Could you check a few things on this drawing? It's one solid part, dimensions in mm from its lowest x, y, z. A direction names the side the tool comes from. Give positions to 0.01 mm unless a question says otherwise; leave off trailing zeros. Write each loop counter-clockwise with the first axis right and the second up, starting at its lowest first coordinate (ties: lowest second). Pieces come first, ordered by that corner, then holes.
1. Suppose I cut it at D-D (y = 26). Please give me the cut outline in (x, z).
2. I'm going to push flat-ended pins straight in: pin 1 (6 mm diameter, centred on y = 37.5, z = 3.5, fed in from -X); pin 2 (1 mm diameter, centred on x = 6, y = 24.5, fed in from +Z); pin 3 (6.5 mm diameter, centred on y = 17, z = 10, fed in from +X). Where does each tip first touch, or does it pass through?
3. Suppose I cut it at C-C (z = 5.75). Please give me the cut outline in (x, y), and give its area (3 significant figures).
4. Thinking about a two-plate mould opening in Y: for the marked faces 5, 6 and 7, which applies, pulls with the +Y half, pulls with the -Y half, needs draft (parallel to the pull), parting line crosses it, or undercut?
5. Suppose I cut it at B-B (z = 9). Please give me the cut outline in (x, y).
6. Suppose I cut it at A-A (x = 5). Please give me the cut outline in (y, z).
7. If I drill on probe 1 along X at (y, z) = (2, 9); probe 2 along Y at (x, z) = (2, 7.5); probe 3 along Z at (x, y) = (25.8, 1.35), over which ranges is the centre line in solid material (lowest first)?
8. On a 3-axis mill with a long thin cutter (end or side, diameter ignored), from which of +Z, -Z, +X, -X, +Y, -Y can I reach the whole of each face in a straight line? I mean the marked faces 1, 2, 3 and 4. Say none if no direction works.
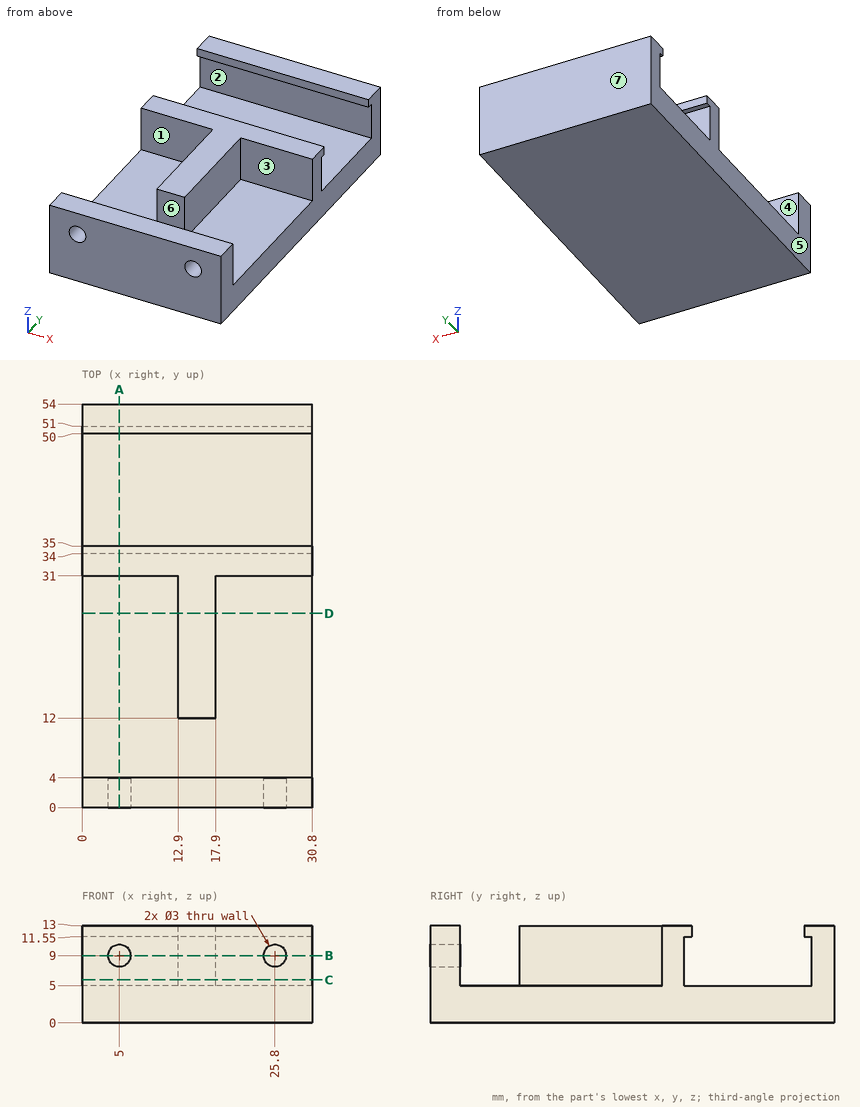
Checks:
1. outline: (0, 0) - (30.8, 0) - (30.8, 5) - (17.9, 5) - (17.9, 13) - (12.9, 13) - (12.9, 5) - (0, 5) - close
2. pin 1: stops at x = 0
2. pin 2: stops at z = 5
2. pin 3: stops at x = 17.9
3. outline: (0, 0) - (30.8, 0) - (30.8, 4) - (0, 4) - close; (0, 31) - (12.9, 31) - (12.9, 12) - (17.9, 12) - (17.9, 31) - (30.8, 31) - (30.8, 34) - (0, 34) - close; (0, 51) - (30.8, 51) - (30.8, 54) - (0, 54) - close
3. area: 403 mm2
4. face 5: needs draft
4. face 6: undercut
4. face 7: pulls with the +Y half
5. outline: (0, 0) - (3.5, 0) - (3.5, 4) - (0, 4) - close; (0, 31) - (12.9, 31) - (12.9, 12) - (17.9, 12) - (17.9, 31) - (30.8, 31) - (30.8, 34) - (0, 34) - close; (0, 51) - (30.8, 51) - (30.8, 54) - (0, 54) - close; (6.5, 0) - (24.3, 0) - (24.3, 4) - (6.5, 4) - close; (27.3, 0) - (30.8, 0) - (30.8, 4) - (27.3, 4) - close
6. outline: (0, 0) - (54, 0) - (54, 13) - (50, 13) - (50, 11.55) - (51, 11.55) - (51, 5) - (34, 5) - (34, 11.55) - (35, 11.55) - (35, 13) - (31, 13) - (31, 5) - (4, 5) - (4, 7.5) - (0, 7.5) - close; (0, 10.5) - (4, 10.5) - (4, 13) - (0, 13) - close
7. probe 1: x = 0 to 3.5, 6.5 to 24.3, 27.3 to 30.8
7. probe 2: y = 0 to 4, 31 to 34, 51 to 54
7. probe 3: z = 0 to 7.5, 10.5 to 13
8. face 1: +Z, -X
8. face 2: +X, -X
8. face 3: +Z, +X
8. face 4: +Z, +X, -X
